```python
from build123d import *

# Parameters (mm, degrees)
SKETCH1_R                = 15
BOSS_EXTRUDE1_DEPTH      = 12
BOSS_EXTRUDE2_DEPTH      = 12
SKETCH3_R                = 4.3
CUT_EXTRUDE1_DEPTH       = 79.135824623
FILLET1_R                = 5
CIRPATTERN1_COUNT        = 3
FILLET1_OF_CIRPATTERN1_R = 5


with BuildPart() as part:
    # Sketch1 → Boss-Extrude1 (new body)
    with BuildSketch(Plane.XY):
        with BuildLine():
            Line((-8.720122643, 33.896304534), (-33.715122143, -9.396304534))
            ThreePointArc((-33.715122143, -9.396304534), (-30.310889132, -17.5), (-24.9949995, -24.5))
            Line((-24.9949995, -24.5), (24.9949995, -24.5))
            ThreePointArc((24.9949995, -24.5), (30.310889132, -17.5), (33.715122143, -9.396304534))
            Line((33.715122143, -9.396304534), (8.720122643, 33.896304534))
            ThreePointArc((8.720122643, 33.896304534), (0, 35), (-8.720122643, 33.896304534))
        make_face()
        Circle(SKETCH1_R, mode=Mode.SUBTRACT)
    extrude(amount=BOSS_EXTRUDE1_DEPTH)

    # Sketch2 → Boss-Extrude2 (add)
    with BuildSketch(Plane(origin=(0, 0, 0), x_dir=(-1, 0, 0), z_dir=(0, 0, -1))):
        Polygon((33.715122143, -9.396304534), (47.571528603, -1.396304534), (42.571528603, 7.263949503), (28.715122143, -0.736050497), align=None)
        Polygon((13.720122643, 25.236050497), (8.720122643, 33.896304534), (22.576529103, 41.896304534), (27.576529103, 33.236050497), align=None)
    boss_extrude2 = extrude(amount=-BOSS_EXTRUDE2_DEPTH)

    # Sketch3 → Cut-Extrude1 (cut, through all)
    with BuildSketch(Plane(origin=(-12.49749975, -21.646304534, 0), x_dir=(0.866025404, -0.5, 0), z_dir=(-0.5, -0.866025404, 0))):
        with Locations((-32.5, 6)):
            Circle(SKETCH3_R)
    cut_extrude1 = extrude(amount=-CUT_EXTRUDE1_DEPTH, mode=Mode.SUBTRACT)

    # Fillet1
    fillet1_edges = [part.edges().sort_by_distance(p)[0] for p in [
        (-45.071528603, 2.933822484, 12),
        (-45.071528603, 2.933822484, 0),
        (-25.076529103, 37.566177516, 12),
        (-25.076529103, 37.566177516, 0),
    ]]
    fillet(fillet1_edges, radius=FILLET1_R)

    # CirPattern1: Boss-Extrude2, Cut-Extrude1 ×3 about axis
    cirpattern1_axis = Axis((0, 0, 0), (0, 0, 1))
    for i in range(1, CIRPATTERN1_COUNT):
        add(boss_extrude2.rotate(cirpattern1_axis, i * 360 / CIRPATTERN1_COUNT))
        add(cut_extrude1.rotate(cirpattern1_axis, i * 360 / CIRPATTERN1_COUNT), mode=Mode.SUBTRACT)

    # Fillet1 of CirPattern1
    fillet1_of_cirpattern1_edges = [part.edges().sort_by_distance(p)[0] for p in [
        (19.9949995, -40.5, 12),
        (19.9949995, -40.5, 0),
        (-19.9949995, -40.5, 12),
        (-19.9949995, -40.5, 0),
        (25.076529103, 37.566177516, 12),
        (25.076529103, 37.566177516, 0),
        (45.071528603, 2.933822484, 12),
        (45.071528603, 2.933822484, 0),
    ]]
    fillet(fillet1_of_cirpattern1_edges, radius=FILLET1_OF_CIRPATTERN1_R)


solid = part.part
```
Could you check a few things on this model? Use its own coordinates, in mm. A direction names the side the tool comes from. Round coordinates to 2 decimals unless told otherwise and drop trailing zeros. Loops run counter-clockwise (first coordinate to the right, second up) from the corner with the lowest first, then second, coordinate; pieces in that order, holes last.
Q1. For P1, Ø4, axis at x = 17.5, z = 2.5, coming from the -Y side; P2, Ø3, axis at y = 4, z = 9, coming from the -X side, each with a flat end and sliding along its axis, tell me the tip position at first contact or that it passes through.
Q2. I want a section at B-B (y = -32.5). Write out the boundary of the cut face in (x, z) (3 decimals).
Q3. On a 3-axis mill with a long thin cutter (end or side, diameter ignored), from which of +Z, -Z, +X, -X, +Y, -Y can I reach the whole of each face in a straight line? I mean faces 4 (the flat face through (14.995, -29, 9)), 5 (the flat face through (37.28, 4.21, 1.92)), 6 (the flat face through (-21.113, 12.432, 5.916)). Say none if no direction works.
Q4. Thinking about a two-plate mould opening in Z: for faces 1 (the cylindrical face through (-30.372, -17.393, 5.916)), 2 (the cylindrical face through (-43.734, 2.243, 1.426)), 3 (the cylindrical face through (20.065, -30.188, 9.626)), which applies, pulls with the +Z half, pulls with the -Z half, needs draft (parallel to the pull), parting line crosses it, or undercut?
Q5. I want a section at C-C (y = 12.5). Write out the boundary of the cut face in (x, z), and give its area (3 significant figures).
Q6. I want a section at A-A (x = 0). Write out the boundary of the cut face in (y, z), and give its area (3 significant figures).
Q7. Please list where these lines run through material, in increasing order: L1, parallel to Z at x = -18, y = -32.5; L2, parallel to X at y = -25, z = 10 (3 decimals); L3, parallel to X at y = -2, z = 10.75.
Answer below:
1. P1: stops at y = -40.47
1. P2: stops at x = -45.02
2. outline: (-24.995, 0) - (-14.995, 0) - (-14.995, 1.7) - (-24.995, 1.7) - close; (-24.995, 10.3) - (-14.995, 10.3) - (-14.995, 12) - (-24.995, 12) - close; (14.995, 0) - (24.995, 0) - (24.995, 1.7) - (14.995, 1.7) - close; (14.995, 10.3) - (24.995, 10.3) - (24.995, 12) - (14.995, 12) - close
3. face 4: +Z, -Z, -Y
3. face 5: +Z, -Z, +Y
3. face 6: +Z, -Z
4. face 1: needs draft
4. face 2: pulls with the -Z half
4. face 3: undercut
5. outline: (-21.07, 0) - (-8.29, 0) - (-8.29, 12) - (-21.07, 12) - close; (8.29, 0) - (21.07, 0) - (21.07, 12) - (8.29, 12) - close
5. area: 307 mm2
6. outline: (-24.5, 0) - (-15, 0) - (-15, 12) - (-24.5, 12) - close; (15, 0) - (35, 0) - (35, 12) - (15, 12) - close
6. area: 354 mm2
7. L1: z = 0 to 1.7, 10.3 to 12
7. L2: x = -24.995 to -14.995, 14.995 to 24.995
7. L3: x = -45.97 to -14.87, 14.87 to 45.97
